```python
from build123d import *

# Parameters (mm, degrees)
SKETCH_W            = 30
SKETCH_H            = 23
PAD002_DEPTH        = 8
POCKET001_DEPTH     = 1.2
SKETCH002_W         = 0.3
SKETCH002_H         = 23
POCKET_DEPTH        = 1
LINEARPATTERN_COUNT = 8
LINEARPATTERN_PITCH = 2.714286


with BuildPart() as part:
    # Sketch → Pad002 (new body)
    with BuildSketch(Plane.XY):
        with Locations((15, 11.5)):
            Rectangle(SKETCH_W, SKETCH_H)
    extrude(amount=PAD002_DEPTH)

    # Sketch001 → Pocket001 (cut)
    with BuildSketch(Plane.XY):
        with BuildLine():
            ThreePointArc((17.966363, 19.115428), (14.961232, 19.899875), (11.966488, 19.07666))
            Line((11.966488, 19.07666), (4.036475, 13.531422))
            ThreePointArc((4.036475, 13.531422), (3.750333, 12.536475), (4, 11.531754))
            Line((4, 11.531754), (12.33, 5.426817))
            ThreePointArc((12.33, 5.426817), (15.374304, 4.811687), (18.318313, 5.80112))
            Line((18.318313, 5.80112), (26, 11.531754))
            ThreePointArc((26, 11.531754), (26.249667, 12.536475), (25.963525, 13.531422))
            Line((25.963525, 13.531422), (17.966363, 19.115428))
        make_face()
    extrude(amount=POCKET001_DEPTH, mode=Mode.SUBTRACT)

    # Sketch002 → Pocket (cut)
    with BuildSketch(Plane.XY):
        with Locations((6.15, 11.5)):
            Rectangle(SKETCH002_W, SKETCH002_H)
    pocket = extrude(amount=POCKET_DEPTH, mode=Mode.SUBTRACT)

    # LinearPattern: Pocket ×8
    with Locations(*[(i * LINEARPATTERN_PITCH, 0, 0) for i in range(1, LINEARPATTERN_COUNT)]):
        add(pocket, mode=Mode.SUBTRACT)


solid = part.part
```
Can you work these out from the model? Positions are in its coordinate system, mm. A direction names the side the tool comes from. Coordinates: 2 decimals unless noted, no trailing zeros. Loops run counter-clockwise (first coordinate to the right, second up) from the corner with the lowest first, then second, coordinate; pieces in that order, holes last.
1) Imagine slicing it at B-B on x = 20.25. List the corners of the cut face in (y, z) for me.
2) I need wall thicknesses on probe 1 along Z at (x, y) = (18.75, 8). Which ranges of the line are inside material? Lowest first, please.
3) Thinking about a two-plate mould opening in Y: for faces 1 (the flat face through (18, 21, 0)), 2 (the flat face through (15, 12, 1.2)), 3 (the flat face through (8.11, 8.52, 0.59)), which applies, pulls with the +Y half, pulls with the -Y half, needs draft (parallel to the pull), parting line crosses it, or undercut?
4) Which directions (+Z, -Z, +X, -X, +Y, -Y) give clear straight access to the entire face, cutting with the end or side of a thin tool? Please do faces 4 (the flat face through (7, 19, 0)), 5 (the flat face through (22.586, 19.4, 0.5)), 6 (the flat face through (22.11, 8.63, 0.59)).
5) Imagine slicing it at A-A on x = 5.25. List the corners of the cut face in (y, z) for me.
Completed:
1. outline: (0, 0) - (7.24, 0) - (7.24, 1.2) - (17.52, 1.2) - (17.52, 0) - (23, 0) - (23, 8) - (0, 8) - close
2. probe 1: z = 1.2 to 8
3. face 1: needs draft
3. face 2: undercut
3. face 3: undercut
4. face 4: -Z, +X, -X, +Y, -Y
4. face 5: -Z, +Y, -Y
4. face 6: -Z
5. outline: (0, 0) - (10.62, 0) - (10.62, 1.2) - (14.38, 1.2) - (14.38, 0) - (23, 0) - (23, 8) - (0, 8) - close
